Geometry check sheet. Reference: the model listing, model coordinates, mm. A direction names the side the tool comes from. Coordinates: 2 decimals unless noted, no trailing zeros. Loops run counter-clockwise (first coordinate to the right, second up) from the corner with the lowest first, then second, coordinate; pieces in that order, holes last. Notation, with made-up numbers: (16, 72.5) - (69, 72.5) arc R12 ccw to (69, 78.5) - close; hole circle Ø7 at (51, 56). An arc over 180 degrees is marked (long way). One line per item, written item: value.
from build123d import *

# Parameters (mm, degrees)
CYLINDER061_R               = 3
CYLINDER061_DEPTH           = 20
CYLINDER060_R               = 3
CYLINDER060_DEPTH           = 30
CYLINDER060_ROLL_ANGLE      = -80.132309
CYLINDER060_PITCH_ANGLE     = -5.803783
CYLINDER060_PLACEMENT_ANGLE = 60.843577


with BuildPart() as cylindre057:
    # Cylinder061 → Cylinder061 (new body)
    with BuildSketch(Plane(origin=(-18, 17, -70), x_dir=(1, 0, 0), z_dir=(0, 0, 1))):
        Circle(CYLINDER061_R)
    extrude(amount=CYLINDER061_DEPTH)


with BuildPart() as fusion030:
    # Cylinder060 → Cylinder060 (new body)
    with BuildSketch(Plane.XY):
        Circle(CYLINDER060_R)
    extrude(amount=CYLINDER060_DEPTH)


with BuildPart() as fusion030_1:
    # Cylinder060 roll: moved
    add(fusion030.part.rotate(Axis((0, 0, 0), (1, 0, 0)), CYLINDER060_ROLL_ANGLE))


with BuildPart() as fusion030_2:
    # Cylinder060 pitch: moved
    add(fusion030_1.part.rotate(Axis((0, 0, 0), (0, 1, 0)), CYLINDER060_PITCH_ANGLE))


with BuildPart() as fusion030_3:
    # Cylinder060 placement: moved
    add(fusion030_2.part.moved(Location((6, 4, -73))).rotate(Axis((6, 4, -73), (0, 0, 1)), CYLINDER060_PLACEMENT_ANGLE))

    # Fusion030: union Cylindre057
    add(cylindre057.part)


solid = fusion030_3.part
(1) Material ranges on probe 1 along X at (y, z) = (8.5, -71); probe 2 along X at (y, z) = (16.75, -57.25); probe 3 along Y at (x, z) = (-13.5, -67), recorded low to high. Write a range as from..to.
Reply:
probe 1: -8.64..3.4
probe 2: -20.99..-15.01
probe 3: 12.27..17.04
(2) Go/stop test with flat-tipped pins: pin 1 Ø1.1 at (x, y) = (-20.5, 18) entering from -Z; pin 2 Ø0.5 at (x, y) = (-19.5, 15) entering from -Z; pin 3 Ø3 at (y, z) = (13.5, -72) entering from -X. Record where each tip stops, or that it passes through.
Reply:
pin 1: z = -70.95
pin 2: z = -70.41
pin 3: x = -17.69
(3) Access from +Z, -Z, +X, -X, +Y, -Y to the whole of each face (thin tool, end or side, straight path). Record for faces 4 (the face through (6, 4, -73)), 5 (the face through (-19.748, 14.562, -69.688)).
Reply:
face 4: -Z, +X, -Y
face 5: -Z, -X, -Y
(4) Cross-section at A-A on z = -64.75. Record the cut outline in (x, y), and give its area (3 significant figures).
Reply:
outline: circle Ø6 at (-18, 17)
area: 28.3 mm2
(5) Release check for a two-part mould opening along Z. For faces 1 (the face through (-20.5, 18.3, -70)), 2 (the face through (-17.1, 19.3, -70)), 3 (the face through (-18, 17, -50)) record: pulls with the +Z half, pulls with the -Z half, needs draft (parallel to the pull), parting line crosses it, or undercut.
Reply:
face 1: undercut
face 2: pulls with the -Z half
face 3: pulls with the +Z half
